Geometry: final body of the model. Coordinates: model frame, mm. A direction names the side the tool comes from. Round coordinates to 2 decimals unless told otherwise and drop trailing zeros. Order: outer loops, then holes, each group sorted by start corner. A loop starts at its lowest first (then second) coordinate and runs counter-clockwise, first axis right, second up. Notation, with made-up numbers: M 41,70 L 99,70 A17 cw 99,102 Z; hole C 13,81.5 d10. An arc over 180 degrees is marked long. Put each result on its own line as item: value. Start each with the question number.
1) Section B-B, the plane x = -81. Return loops of the section in (y, z), then the cut area to 3 significant figures.
2) Material intervals for probe 1 along Y at (x, z) = (-81.5, -31); probe 2 along Z at (x, y) = (-77.5, -156.5); probe 3 along Y at (x, z) = (-78, -49), sorted ascending. Write a range as [from, to].
3) First-contact query: P1, Ø1.5, axis at x = -85.5, y = -102.5, coming from the -Z side; P2, Ø3.5, axis at y = -180, z = 26, coming from the +X side; P3, Ø5, axis at x = -85, z = 46, coming from the +Y side. Flat tips, straight axial feed; report the tip coordinate or a pass-through.
4) Access query for faces 1 (the cylindrical face through (-82.4, -7.4, 86.2)), 2 (the cylindrical face through (-81.2, -180.5, -60)), 3 (the cylindrical face through (-81.142, -170.003, -0.771)). Directions: +Z, -Z, +X, -X, +Y, -Y. A direction counts if a zero-diameter tool reaches every point of the face in a straight line with its end or side. Return the directions, or none.
5) Section A-A, the plane z = -23. Return loops of the section in (x, y).
from build123d import *

# Parameters (mm, degrees)
SKETCH4_R                = 5
BOSS_EXTRUDE2_DEPTH      = 56
BOSS_EXTRUDE2_DEPTH_BACK = 56
SKETCH5_W                = 8
SKETCH5_H                = 3
SKETCH6_W                = 4
SKETCH6_H                = 3
REVOLVE1_ANGLE           = 180


with BuildPart() as part:
    # Sweep7: sweep along a path in Sketch2
    with BuildLine(Plane(origin=(-81.317279836, 0, 0), x_dir=(0, 0, -1), z_dir=(1, 0, 0))) as sweep7_path:
        Line((0, -175), (-55.045760302, -175))
        ThreePointArc((-55.045760302, -175), (-65.230021906, -171.012756947), (-70, -161.170775411))
        Line((-70, -161.170775411), (-81.191157553, -18.226833323))
        ThreePointArc((-81.191157553, -18.226833323), (-81.285737233, -16.614648578), (-81.317279836, -15))
        Line((-81.317279836, -15), (-81.317279836, 0))
    # Sketch4 → Sweep7 (sweep)
    with BuildSketch(Plane.XY):
        with Locations((-81.317279836, -175)):
            Circle(SKETCH4_R)
    sweep7 = sweep(path=sweep7_path.line)

    # Mirror2: Sweep7 across plane
    add(sweep7.mirror(Plane.XY))

    # Sketch5 → Boss-Extrude2 (add, two sides: drawn at the far end of the back side and taken through both)
    with BuildSketch(Plane.XY.offset(-BOSS_EXTRUDE2_DEPTH_BACK)):
        with Locations((-81.317279836, -180.5)):
            Rectangle(SKETCH5_W, SKETCH5_H)
    extrude(amount=BOSS_EXTRUDE2_DEPTH + BOSS_EXTRUDE2_DEPTH_BACK)

    # Sketch6 → Revolve1 (revolve)
    with BuildSketch(Plane.XY.offset(56)):
        with Locations((-79.317279836, -180.5)):
            Rectangle(SKETCH6_W, SKETCH6_H)
    revolve1 = revolve(axis=Axis((-81.317279836, -182, 56), (0, -1, 0)), revolution_arc=REVOLVE1_ANGLE)

    # Mirror3: Revolve1 across plane
    add(revolve1.mirror(Plane.XY))


solid = part.part
Result sheet:
1. outline: M -182,-59.99 L -179.37,-59.99 A19.99 ccw -161.56,-74.97 L -18.62,-86.17 A46.33 ccw -15,-86.31 L 0,-86.31 L 0,-76.33 L -15,-76.33 A36.35 cw -17.84,-76.22 L -160.78,-65.03 A10.01 cw -170.01,-55.05 L -170.01,55.05 A10.01 cw -160.78,65.03 L -17.84,76.22 A36.35 cw -15,76.33 L 0,76.33 L 0,86.31 L -15,86.31 A46.33 ccw -18.62,86.17 L -161.56,74.97 A19.99 ccw -179.37,59.99 L -182,59.99 Z
1. area: 5,010 mm2
2. probe 1: y = [-182, -170]
2. probe 2: z = [-73.6, -67.13], [67.13, 73.6]
2. probe 3: y = [-182, -179], [-178.74, -171.26]
3. P1: stops at z = -78.24
3. P2: stops at x = -77.32
3. P3: stops at y = -170.14
4. face 1: +Y
4. face 2: -Z, -Y
4. face 3: none
5. outline: M -85.32,-182 L -77.32,-182 L -77.32,-179 L -78.32,-179 A5 ccw long -84.32,-179 L -85.32,-179 Z
